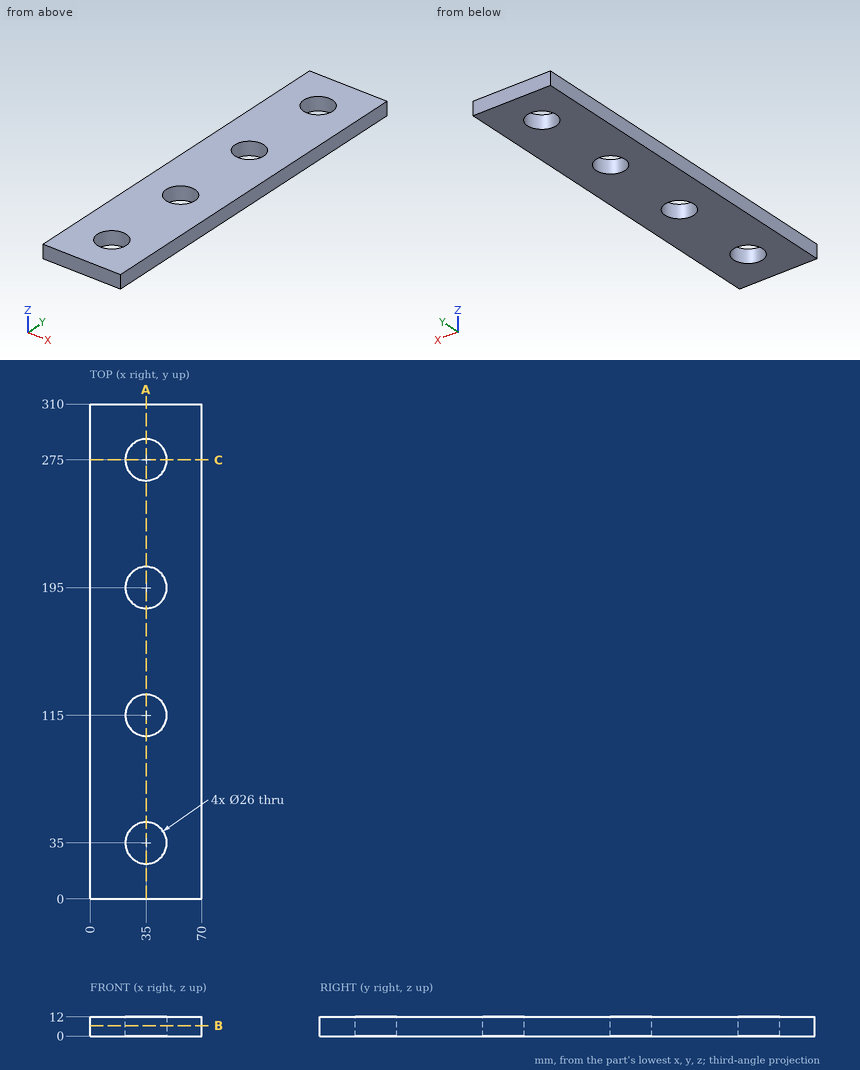
Study the drawing (mm; zero at the part's minimum x, y, z) and answer. Round coordinates to 2 decimals unless told otherwise and drop trailing zeros. Write each loop counter-clockwise with the first axis right and the second up, starting at its lowest first coordinate (ties: lowest second). Pieces come first, ordered by that corner, then holes.
1) A cutting plane is placed at A-A on x = 35. Determine the outline of the cut face in (y, z), and give its area (3 significant figures).
2) A cutting plane is placed at B-B on z = 6.5. Determine the outline of the cut face in (x, y).
3) A flat-ended cylindrical pin translates along its axis: P1, Ø21, axis at x = 35, y = 115, coming from the -Z side. Find the tip coordinate at first contact, or state that the pin passes through.
4) A cutting plane is placed at C-C on y = 275. Determine the outline of the cut face in (x, z).
5) Consider probe 1 along Y at (x, z) = (35, 7.5); probe 2 along X at (y, z) = (276, 10.5); probe 3 along Y at (x, z) = (30.5, 5.75). Determine where each line is inside the solid, lowest interval first.
Entries:
1. outline: (0, 0) - (22, 0) - (22, 12) - (0, 12) - close; (48, 0) - (102, 0) - (102, 12) - (48, 12) - close; (128, 0) - (182, 0) - (182, 12) - (128, 12) - close; (208, 0) - (262, 0) - (262, 12) - (208, 12) - close; (288, 0) - (310, 0) - (310, 12) - (288, 12) - close
1. area: 2,470 mm2
2. outline: (0, 0) - (70, 0) - (70, 310) - (0, 310) - close; hole circle Ø26 at (35, 35); hole circle Ø26 at (35, 115); hole circle Ø26 at (35, 195); hole circle Ø26 at (35, 275)
3. P1: passes through
4. outline: (0, 0) - (22, 0) - (22, 12) - (0, 12) - close; (48, 0) - (70, 0) - (70, 12) - (48, 12) - close
5. probe 1: y = 0 to 22, 48 to 102, 128 to 182, 208 to 262, 288 to 310
5. probe 2: x = 0 to 22.04, 47.96 to 70
5. probe 3: y = 0 to 22.8, 47.2 to 102.8, 127.2 to 182.8, 207.2 to 262.8, 287.2 to 310
